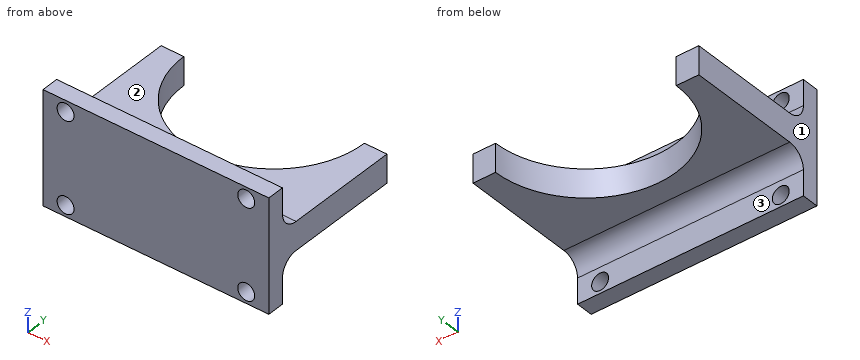
```python
from build123d import *

# Parameters (mm, degrees)
BOSS_EXTRUDE1_DEPTH      = 2.5
BOSS_EXTRUDE1_DEPTH_BACK = 2.5
SKETCH1_W                = 40
SKETCH1_H                = 26
SKETCH2_R                = 16
CUT_EXTRUDE1_DEPTH       = 25.372115214
BOSS_EXTRUDE2_DEPTH      = 10
BOSS_EXTRUDE2_DEPTH_BACK = 10
SKETCH3_W                = 40
SKETCH3_H                = 3
FILLET1_R                = 3
SKETCH4_R                = 1.5
CUT_EXTRUDE2_DEPTH       = 33.078029865
MIRROR2_COPY_1_SKETCH_R  = 1.5
MIRROR2_COPY_1_DEPTH     = 33.078029865


with BuildPart() as part:
    # Sketch1 → Boss-Extrude1 (new, two sides: drawn at the far end of the back side and taken through both)
    with BuildSketch(Plane.XY.offset(-BOSS_EXTRUDE1_DEPTH_BACK)):
        Rectangle(SKETCH1_W, SKETCH1_H)
    extrude(amount=BOSS_EXTRUDE1_DEPTH + BOSS_EXTRUDE1_DEPTH_BACK)

    # Sketch2 → Cut-Extrude1 (cut, through all)
    with BuildSketch(Plane(origin=(0, 0, -2.5), x_dir=(-1, 0, 0), z_dir=(0, 0, -1))):
        with Locations((0, 13)):
            Circle(SKETCH2_R)
    extrude(amount=-CUT_EXTRUDE1_DEPTH, mode=Mode.SUBTRACT)

    # Sketch3 → Boss-Extrude2 (add, two sides: drawn at the far end of the back side and taken through both)
    with BuildSketch(Plane.XY.offset(-BOSS_EXTRUDE2_DEPTH_BACK)):
        with Locations((0, -11.5)):
            Rectangle(SKETCH3_W, SKETCH3_H)
    extrude(amount=BOSS_EXTRUDE2_DEPTH + BOSS_EXTRUDE2_DEPTH_BACK)

    # Fillet1
    fillet1_edges = [part.edges().sort_by_distance(p)[0] for p in [
        (0, -10, 2.5),
        (0, -10, -2.5),
    ]]
    fillet(fillet1_edges, radius=FILLET1_R)

    # Sketch4 → Cut-Extrude2 (cut, through all)
    with BuildSketch(Plane(origin=(0, -10, 0), x_dir=(1, 0, 0), z_dir=(0, 1, 0))):
        with Locations(Location((16, 8, 0), (0, 0, 270))):
            Circle(SKETCH4_R)
    cut_extrude2 = extrude(amount=-CUT_EXTRUDE2_DEPTH, mode=Mode.SUBTRACT)

    # Mirror1: Cut-Extrude2 across plane
    add(cut_extrude2.mirror(Plane.XY), mode=Mode.SUBTRACT)

    # Mirror2: Cut-Extrude2 across plane
    add(cut_extrude2.mirror(Plane(origin=(0, 0, 0), x_dir=(0, 0, 1), z_dir=(1, 0, 0))), mode=Mode.SUBTRACT)

    # Mirror2 copy 1 sketch → Mirror2 copy 1 (cut, through all)
    with BuildSketch(Plane(origin=(0, -10, 0), x_dir=(-1, 0, 0), z_dir=(0, 1, 0))):
        with Locations(Location((16, 8, 0), (0, 0, 270))):
            Circle(MIRROR2_COPY_1_SKETCH_R)
    extrude(amount=-MIRROR2_COPY_1_DEPTH, mode=Mode.SUBTRACT)


solid = part.part
```
Here's how the part is built. I have some questions about the finished solid (model axes, mm). Face numbers are marked on the shaded views. A direction names the side the tool comes from. Coordinates: 2 decimals unless noted, no trailing zeros. Write each loop counter-clockwise with the first axis right and the second up, starting at its lowest first coordinate (ties: lowest second). Pieces come first, ordered by that corner, then holes. Notation, with made-up numbers: (69.5, 81) -> (78.5, 81) arc R16 ccw to (78.5, 89) -> close; hole circle Ø5 at (12.25, -5.75). An arc over 180 degrees is marked (long way). Use a Markdown table: item, result. Add a question column.
(1) I'm going to push flat-ended pins straight in: P1, Ø1.3, axis at x = -9, z = 6.5, coming from the +Y side; P2, Ø6, axis at x = 10, y = 4, coming from the -Z side; P3, Ø10, axis at x = -6, z = 5, coming from the +Y side. Where does each tip first touch, or does it pass through?
(2) Please list where these lines run through material, in increasing order: line 1 (Z direction, x = -16, y = -11.2); line 2 (X direction, y = -11.55, z = -8); line 3 (Z direction, x = 13.5, y = 1.5).
(3) If we section it at D-D, the plane z = -1: Write out the boundary of the cut face in (x, y).
(4) If we section it at B-B, the plane x = 0: Write out the boundary of the cut face in (y, z).
(5) If we section it at A-A, the plane z = 8: Write out the boundary of the cut face in (x, y).
(6) For the marked faces 1, 2 and 3, which set-ups out of +Z, -Z, +X, -X, +Y, -Y let a thin tool reach every point of the face, with its end or its side?
(7) If we section it at C-C, the plane y = 6.75: Write out the boundary of the cut face in (x, z).
Outcome:
| question | item | result |
|---|---|---|
| 1 | P1 | stops at y = -10 |
| 1 | P2 | stops at z = -2.5 |
| 1 | P3 | stops at y = 0.78 |
| 2 | line 1 | z = -10 to -9.5, -6.5 to 6.5, 9.5 to 10 |
| 2 | line 2 | x = -20 to -17.5, -14.5 to 14.5, 17.5 to 20 |
| 2 | line 3 | z = -2.5 to 2.5 |
| 3 | outline | (-20, -13) -> (20, -13) -> (20, 13) -> (16, 13) arc R16 cw to (-16, 13) -> (-20, 13) -> close |
| 4 | outline | (-13, -10) -> (-10, -10) -> (-10, -5.5) arc R3 cw to (-7, -2.5) -> (-3, -2.5) -> (-3, 2.5) -> (-7, 2.5) arc R3 cw to (-10, 5.5) -> (-10, 10) -> (-13, 10) -> close |
| 5 | outline | (-20, -13) -> (-17.5, -13) -> (-17.5, -10) -> (-20, -10) -> close; (-14.5, -13) -> (14.5, -13) -> (14.5, -10) -> (-14.5, -10) -> close; (17.5, -13) -> (20, -13) -> (20, -10) -> (17.5, -10) -> close |
| 6 | face 1 | +Z, -Z, -X, +Y, -Y |
| 6 | face 2 | +Z, +X, -X, +Y |
| 6 | face 3 | -Z, +X, -X, +Y |
| 7 | outline | (-20, -2.5) -> (-14.73, -2.5) -> (-14.73, 2.5) -> (-20, 2.5) -> close; (14.73, -2.5) -> (20, -2.5) -> (20, 2.5) -> (14.73, 2.5) -> close |
